Could you check a few things on this model? Use its own coordinates, in mm. Face numbers are marked on the shaded views. A direction names the side the tool comes from. Give positions to 0.01 mm unless a question says otherwise; leave off trailing zeros. Write each loop counter-clockwise with the first axis right and the second up, starting at its lowest first coordinate (ties: lowest second). Pieces come first, ordered by that corner, then holes. Notation, with made-up numbers: M 72.5,57 L 76.5,57 A20 cw 76.5,93 Z; hole C -25,16 d2. An arc over 180 degrees is marked long. Answer as a JSON object with one key per item and string values. Group by question number.
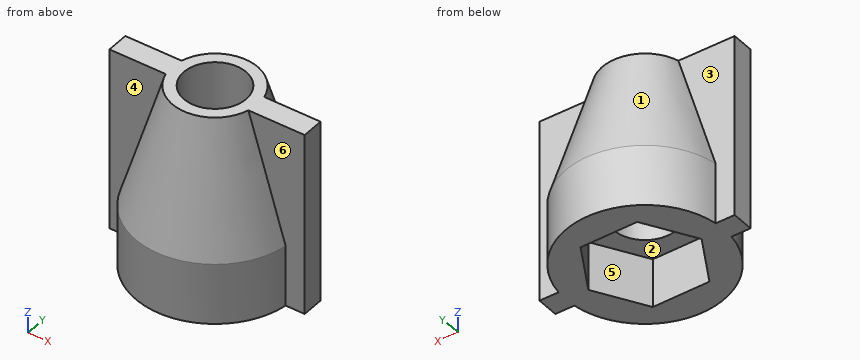
```python
from build123d import *

# Parameters (mm, degrees)
F0_R     = 6.5
F1_DEPTH = 15
F2_SIZE2 = 10
F2_SIZE  = 3
F3_W     = 16
F3_H     = 1.8
F4_DEPTH = 15
F6_DEPTH = 4
F7_R     = 2.55
F8_DEPTH = 25


with BuildPart() as f1:
    # F0 (on Top) → F1 (new body)
    with BuildSketch(Plane.XY):
        Circle(F0_R)
    extrude(amount=F1_DEPTH)

    # F2
    f2_edges = [f1.edges().sort_by_distance(p)[0] for p in [
        (-6.5, 0, 15),
    ]]
    f2_side = f1.faces().sort_by_distance((0, 0, 15))[0]
    chamfer(f2_edges, length=F2_SIZE, length2=F2_SIZE2, reference=f2_side)

    # F3 (on face) → F4 (join)
    with BuildSketch(Plane.XY.offset(15)):
        Rectangle(F3_W, F3_H)
    extrude(amount=-F4_DEPTH)

    # F5 (on face) → F6 (cut)
    with BuildSketch(Plane(origin=(0, 0, 0), x_dir=(1, 0, 0), z_dir=(0, 0, -1))):
        Polygon((2.3803777429, -4.0253946143), (4.6762828677, 0.0487702888), (2.2959051248, 4.0741649031), (-2.3803777429, 4.0253946143), (-4.6762828677, -0.0487702888), (-2.2959051248, -4.0741649031), align=None)
    extrude(amount=-F6_DEPTH, mode=Mode.SUBTRACT)

    # F7 (on face) → F8 (cut)
    with BuildSketch(Plane.XY.offset(15)):
        Circle(F7_R)
    extrude(amount=-F8_DEPTH, mode=Mode.SUBTRACT)


solid = f1.part
```
1) If we section it at A-A, the plane z = 3.25: List the corners of the cut face in (x, y) for me.
2) If we section it at B-B, the plane x = 0: List the corners of the cut face in (y, z) for me, plus the area to 3 significant figures.
3) I'm going to push flat-ended pins straight in: pin 1 (2.5 mm diameter, centred on x = -5, z = 9, fed in from -Y); pin 2 (5 mm diameter, centred on x = 5.5, z = 4.5, fed in from -Y); pin 3 (1.4 mm diameter, centred on x = -6, z = 9, fed in from +Y). Where does each tip first touch, or does it pass through?
4) For the marked faces 4, 5 and 6, which set-ups out of +Z, -Z, +X, -X, +Y, -Y let a thin tool reach every point of the face, with its end or its side?
5) If we section it at D-D, the plane z = 10.75: List the corners of the cut face in (x, y) for me (3 decimals), plus the area to 3 significant figures.
6) We'd pull the mould along X, two halves only. Please class the marked faces 1, 2 and 3: released by +X, released by -X, zero draft, split by the parting line, or undercut.
7) Please list where these lines run through material, in increasing order: line 1 along Y through (x, z) = (-6, 9); line 2 along Z through (x, y) = (2.25, 2); line 3 along X through (y, z) = (0.25, 14.25). Write a range as from..to.
8) If we section it at C-C, the plane x = -7: List the corners of the cut face in (y, z) for me.
Taken from the geometry:
{
 "1": {"outline": "M -8,-0.9 L -6.44,-0.9 A6.5 ccw 6.44,-0.9 L 8,-0.9 L 8,0.9 L 6.44,0.9 A6.5 ccw -6.44,0.9 L -8,0.9 Z; hole M -4.68,0.05 L -2.38,-4.03 L 2.3,-4.07 L 4.68,-0.05 L 2.38,4.03 L -2.3,4.07 Z"},
 "2": {"outline": "M -6.5,0 L -4.05,0 L -4.05,4 L -2.55,4 L -2.55,15 L -3.5,15 L -6.5,5 Z; M 2.55,4 L 4.05,4 L 4.05,0 L 6.5,0 L 6.5,5 L 3.5,15 L 2.55,15 Z", "area": "76.5 mm²"},
 "3": {"pin 1": "y = -3.85", "pin 2": "y = -5.77", "pin 3": "y = 0.9"},
 "4": {"face 4": "+Z, -X, -Y", "face 5": "-Z", "face 6": "+Z, +X, -Y"},
 "5": {"outline": "M -8,-0.9 L -4.689,-0.9 A4.775 ccw 4.689,-0.9 L 8,-0.9 L 8,0.9 L 4.689,0.9 A4.775 ccw -4.689,0.9 L -8,0.9 Z; hole C 0,0 d5.1", "area": "62.9 mm²"},
 "6": {"face 1": "split by the parting line", "face 2": "undercut", "face 3": "zero draft"},
 "7": {"line 1": "-0.9..0.9", "line 2": "4..15", "line 3": "-8..-2.54, 2.54..8"},
 "8": {"outline": "M -0.9,0 L 0.9,0 L 0.9,15 L -0.9,15 Z"}
}
